from build123d import *

# Parameters (mm, degrees)
SKETCH1_R               = 3
BOSS_EXTRUDE1_DEPTH     = 23.5
CUT_EXTRUDE1_DEPTH      = 24.879907873
CUT_EXTRUDE1_DEPTH_BACK = 24.879907873
SKETCH2_R               = 1.5
CUT_EXTRUDE2_DEPTH      = 24.879907996
CUT_EXTRUDE2_DEPTH_BACK = 24.879907996
SKETCH3_R               = 1.5


with BuildPart() as part:
    # Sketch1 → Boss-Extrude1 (new, symmetric)
    with BuildSketch(Plane.YZ):
        with Locations(Location((0, 0, 0), (0, 0, 270))):
            Circle(SKETCH1_R)
    extrude(amount=BOSS_EXTRUDE1_DEPTH, both=True)

    # Sketch2 → Cut-Extrude1 (cut, two sides: drawn at the far end of the back side and taken through both)
    with BuildSketch(Plane(origin=(0, 0, 0), x_dir=(0, 1, 0), z_dir=(0, 0, 1)).offset(-CUT_EXTRUDE1_DEPTH_BACK)):
        with Locations(Location((0, -11.5, 0), (0, 0, 270))):
            Circle(SKETCH2_R)
    extrude(amount=CUT_EXTRUDE1_DEPTH + CUT_EXTRUDE1_DEPTH_BACK, mode=Mode.SUBTRACT)

    # Sketch3 → Cut-Extrude2 (cut, two sides: drawn at the far end of the back side and taken through both)
    with BuildSketch(Plane(origin=(0, 0, 0), x_dir=(-1, 0, 0), z_dir=(0, 0.8660254037844364, -0.5000000000000041)).offset(-CUT_EXTRUDE2_DEPTH_BACK)):
        with Locations(Location((11.5, 0, 0), (0, 0, 90))):
            Circle(SKETCH3_R)
    extrude(amount=CUT_EXTRUDE2_DEPTH + CUT_EXTRUDE2_DEPTH_BACK, mode=Mode.SUBTRACT)


solid = part.part
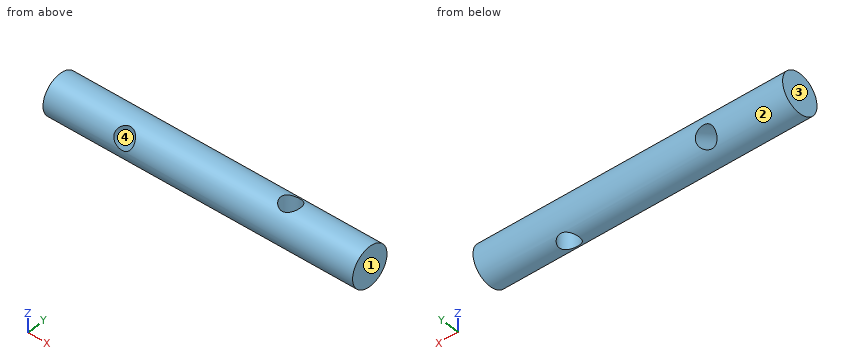
Here's how the part is built. I have some questions about the finished solid (model axes, mm). Face numbers are marked on the shaded views. Round coordinates to 2 decimals unless told otherwise and drop trailing zeros. Order: outer loops, then holes, each group sorted by start corner. A loop starts at its lowest first (then second) coordinate and runs counter-clockwise, first axis right, second up. Notation, with made-up numbers: (83, -2.5) -> (89, -2.5) arc R29 cw to (89, 29.5) -> close; hole circle Ø1 at (80, -23). An arc over 180 degrees is marked (long way). Use CSV: the item, a comma, the result in double quotes.
1. I want a section at C-C on x = -8. List the corners of the cut face in (y, z) for me, and give its area (3 significant figures).
Recorded:
outline,"circle Ø6 at (0, 0)"
area,"28.3 mm2"
2. I want a section at B-B on y = 0.5. Give the number of separate pieces and of enclosed holes in the cut face, and give its area (3 significant figures).
Recorded:
separate pieces,"2"
enclosed holes,"1"
area,"253 mm2"
3. I need wall thicknesses on line 1 along X through (y, z) = (0, 0); line 2 along X through (y, z) = (-0.25, 1); line 3 along Z through (x, y) = (4, 0.25). Which ranges of each line are inside material? Lowest first, please.
Recorded:
line 1,"x = -23.5 to -13, -10 to 10, 13 to 23.5"
line 2,"x = -23.5 to -12.8, -10.2 to 10.02, 12.98 to 23.5"
line 3,"z = -2.99 to 2.99"
4. I want a section at A-A on x = 11.5. List the corners of the cut face in (y, z) for me.
Recorded:
outline,"(-1.5, -2.6) -> (-1.5, 2.6) arc R3 ccw to start; (1.5, -2.6) arc R3 ccw to (1.5, 2.6) -> close"
5. Thinking about a two-plate mould opening in X: for the marked faces 1, 2, 3 and 4, which applies, pulls with the +X half, pulls with the -X half, needs draft (parallel to the pull), parting line crosses it, or undercut?
Recorded:
face 1,"pulls with the +X half"
face 2,"needs draft"
face 3,"pulls with the -X half"
face 4,"undercut"
6. I'm going to push flat-ended pins straight in: P1, Ø2.5, axis at x = 11.5, y = 0, coming from the -Z side; P2, Ø2, axis at x = -17, z = 1.5, coming from the -Y side. Where does each tip first touch, or does it pass through?
Recorded:
P1,"passes through"
P2,"stops at y = -2.96"
